CAD build for the part. Positions are in the model's coordinates, mm. Face numbers are marked on the shaded views. A direction names the side the tool comes from. Round coordinates to 2 decimals unless told otherwise and drop trailing zeros. Order: outer loops, then holes, each group sorted by start corner. A loop starts at its lowest first (then second) coordinate and runs counter-clockwise, first axis right, second up. Notation, with made-up numbers: (59, 37.25) -> (105, 37.25) arc R17 ccw to (105, 67.25) -> close; hole circle Ø7 at (71, 10.5). An arc over 180 degrees is marked (long way). Return JSON: item names as keys, results as strings. Group by question number.
Q1. Cut at B-B (x = 18.5). Write the cut outline in (y, z).
Q2. Flat gauge pins, fed straight in: pin 1 (4 mm diameter, centred on y = 13, z = 17.5, fed in from -X); pin 2 (6.5 mm diameter, centred on x = -7, z = 25.5, fed in from -Y); pin 3 (4 mm diameter, centred on x = 28.5, z = 26.5, fed in from -Y). Where does each tip first touch, or does it go through?
Q3. Which spindle directions (+Z, -Z, +X, -X, +Y, -Y) get a long thin tool onto all of the face, cutting with end or side? Do the marked faces 4, 5 and 6. Say none if no direction does.
Q4. Mould opens along Y. For the marked faces 1, 2 and 3 say: +Y half, -Y half, draft (parallel to the pull), parting line (faces both ways), or undercut.
Q5. Cut at A-A (y = 0). Write the cut outline in (x, z), then the cut area to 3 significant figures.
Q6. Cut at D-D (x = -4). Count the separate pieces of the cut face and the enclosed holes in it, then the cut area to 3 significant figures.
Q7. Probe line 1 along Y through (x, z) = (0, 29); line 2 along Y through (x, z) = (0, 54); line 3 along Z through (x, y) = (4.5, -5). List the from-to ranges inside material, lowest first.
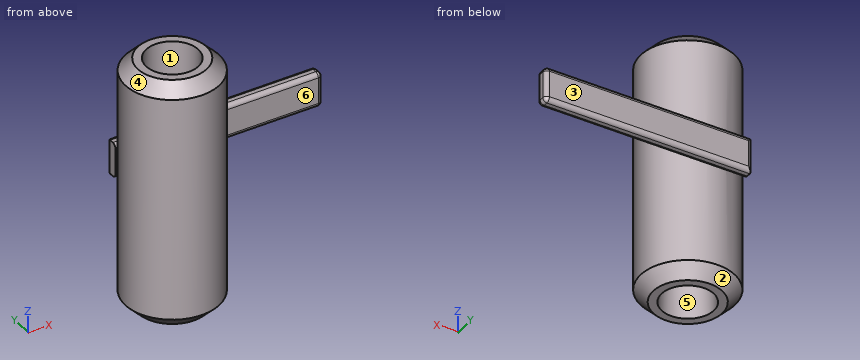
from build123d import *

# Parameters (mm, degrees)
F0_R          = 7.9375
F0_R_2        = 6.35
F2_DEPTH      = 50.8
F3_R          = 14.2875
F3_R_2        = 7.9375
F4_DEPTH      = 63.5
F4_DEPTH_BACK = 12.7
F5_SIZE       = 3.81
F7_START      = -13.97
F6_W          = 64.1522035003
F6_H          = 10.4847997427
F7_DEPTH      = 3.81
F8_T1_DEPTH   = 66.0572035003
F8_T3_DEPTH   = 16.8347997427
F8_T5_DEPTH   = 7.9447997427
F8_T7_DEPTH   = 1.27
F8_S11_W      = 1.27
F8_S11_H      = 1.27
F8_T12_DEPTH  = 1.27
F8_S17_W      = 1.27
F8_S17_H      = 1.27
F8_T18_DEPTH  = 1.27
F8_S23_W      = 1.27
F8_S23_H      = 1.27
F8_T24_DEPTH  = 1.27
F8_S29_W      = 1.27
F8_S29_H      = 1.27
F8_T30_DEPTH  = 1.27
F8_T36_DEPTH  = 54.3607688419
F8_S37_R      = 14.2875
F8_T38_DEPTH  = 29
F8_T42_DEPTH  = 54.3607688419
F8_S43_R      = 14.2875
F8_T44_DEPTH  = 29
F8_T48_DEPTH  = 12.0558566395
F8_S49_R      = 14.2875
F8_T50_DEPTH  = 8
F8_T54_DEPTH  = 12.0558566395
F8_S55_R      = 14.2875
F8_T56_DEPTH  = 8


# Not quite as in the source:
# - a fillet or chamfer that OpenCascade refuses, or shapes differently, is made with other operations: its cross-section is extruded or revolved along the edge and cut away or added
# - a feature names something its author has since deleted; it is built from what else it names


with BuildPart() as f2:
    # F0 (on Top) → F2 (new body)
    with BuildSketch(Plane.XY):
        Circle(F0_R)
        Circle(F0_R_2, mode=Mode.SUBTRACT)
    extrude(amount=F2_DEPTH)

    # F3 (on face) → F4 (join, two sides)
    with BuildSketch(Plane.XY) as f4_sk:
        Circle(F3_R)
        Circle(F3_R_2, mode=Mode.SUBTRACT)
    extrude(amount=F4_DEPTH)
    extrude(f4_sk.sketch, amount=-F4_DEPTH_BACK)

    # F5
    f5_edges = [f2.edges().sort_by_distance(p)[0] for p in [
        (-14.2875, 0, 63.5),
        (-14.2875, 0, -12.7),
    ]]
    chamfer(f5_edges, length=F5_SIZE)

    # F6 (on Front) → F7 (join)
    with BuildSketch(Plane.XZ.offset(F7_START)):
        with Locations((23.3749561012, 26.5372619033)):
            Rectangle(F6_W, F6_H)
    extrude(amount=-F7_DEPTH)

    # F8: fillet of radius 1.27 on 11 edges, made by hand

    # F8_s2 → F8_t1 (cut)
    with BuildSketch(Plane.YZ.offset(-11.876145649)):
        with BuildLine():
            ThreePointArc((16.51, 31.7796617746), (17.4080256121, 31.4076873867), (17.78, 30.5096617746))
            Line((17.78, 30.5096617746), (17.78, 31.7796617746))
            Line((17.78, 31.7796617746), (16.51, 31.7796617746))
        make_face()
        with BuildLine():
            ThreePointArc((16.51, 21.2948620319), (17.4080256121, 21.6668364198), (17.78, 22.5648620319))
            Line((17.78, 22.5648620319), (17.78, 21.2948620319))
            Line((17.78, 21.2948620319), (16.51, 21.2948620319))
        make_face()
    extrude(amount=F8_T1_DEPTH, mode=Mode.SUBTRACT)

    # F8_s4 → F8_t3 (cut)
    with BuildSketch(Plane.XY.offset(18.1198620319)):
        with BuildLine():
            ThreePointArc((-7.431145649, 17.78), (-8.3291712611, 17.4080256121), (-8.701145649, 16.51))
            Line((-8.701145649, 16.51), (-8.701145649, 17.78))
            Line((-8.701145649, 17.78), (-7.431145649, 17.78))
        make_face()
    extrude(amount=F8_T3_DEPTH, mode=Mode.SUBTRACT)

    # F8_s6 → F8_t5 (cut)
    with BuildSketch(Plane.XY.offset(22.5648620319)):
        with BuildLine():
            ThreePointArc((54.1810578513, 13.97), (55.0790834634, 14.3419743879), (55.4510578513, 15.24))
            Line((55.4510578513, 15.24), (55.4510578513, 13.97))
            Line((55.4510578513, 13.97), (54.1810578513, 13.97))
        make_face()
        with BuildLine():
            ThreePointArc((55.4510578513, 16.51), (55.0790834634, 17.4080256121), (54.1810578513, 17.78))
            Line((54.1810578513, 17.78), (55.4510578513, 17.78))
            Line((55.4510578513, 17.78), (55.4510578513, 16.51))
        make_face()
    extrude(amount=F8_T5_DEPTH, mode=Mode.SUBTRACT)

    # F8_s8 → F8_t7 (cut)
    with BuildSketch(Plane.XZ.offset(-16.51)):
        with BuildLine():
            ThreePointArc((54.1810578513, 31.7796617746), (55.0790834634, 31.4076873867), (55.4510578513, 30.5096617746))
            Line((55.4510578513, 30.5096617746), (55.4510578513, 31.7796617746))
            Line((55.4510578513, 31.7796617746), (54.1810578513, 31.7796617746))
        make_face()
        with BuildLine():
            ThreePointArc((54.1810578513, 21.2948620319), (55.0790834634, 21.6668364198), (55.4510578513, 22.5648620319))
            Line((55.4510578513, 22.5648620319), (55.4510578513, 21.2948620319))
            Line((55.4510578513, 21.2948620319), (54.1810578513, 21.2948620319))
        make_face()
    extrude(amount=F8_T7_DEPTH, mode=Mode.SUBTRACT)


with BuildPart() as f8_tool10:
    # F8_s11 → F8_t12 (new body)
    with BuildSketch(Plane.XY.offset(30.5096617746)):
        with Locations((54.8160578513, 17.145)):
            Rectangle(F8_S11_W, F8_S11_H)
    extrude(amount=F8_T12_DEPTH)

    # F8_s13 → F8_t14 (revolve, cut)
    with BuildSketch(Plane(origin=(54.1810578513, 16.51, 30.5096617746), x_dir=(-0.7071067812, -0.7071067812, 0), z_dir=(-0.7071067812, 0.7071067812, 0))):
        with BuildLine():
            ThreePointArc((0, -1.27), (1.27, 0), (0, 1.27))
            Line((0, 1.27), (0, -1.27))
        make_face()
    revolve(axis=Axis((54.1810578513, 16.51, 30.5096617746), (0, 0, 1)), mode=Mode.SUBTRACT)


with BuildPart() as f2_1:
    add(f2.part)

    # F8_t9: cut F8_tool10
    add(f8_tool10.part, mode=Mode.SUBTRACT)


with BuildPart() as f8_tool16:
    # F8_s17 → F8_t18 (new body)
    with BuildSketch(Plane.YZ.offset(54.1810578513)):
        with Locations((17.145, 21.9298620319)):
            Rectangle(F8_S17_W, F8_S17_H)
    extrude(amount=F8_T18_DEPTH)

    # F8_s19 → F8_t20 (revolve, cut)
    with BuildSketch(Plane(origin=(54.1810578513, 16.51, 22.5648620319), x_dir=(0, -0.7071067812, 0.7071067812), z_dir=(0, 0.7071067812, 0.7071067812))):
        with BuildLine():
            ThreePointArc((0, -1.27), (1.27, 0), (0, 1.27))
            Line((0, 1.27), (0, -1.27))
        make_face()
    revolve(axis=Axis((54.1810578513, 16.51, 22.5648620319), (1, 0, 0)), mode=Mode.SUBTRACT)


with BuildPart() as f2_2:
    add(f2_1.part)

    # F8_t15: cut F8_tool16
    add(f8_tool16.part, mode=Mode.SUBTRACT)


with BuildPart() as f8_tool22:
    # F8_s23 → F8_t24 (new body)
    with BuildSketch(Plane.YZ.offset(54.1810578513)):
        with Locations((14.605, 21.9298620319)):
            Rectangle(F8_S23_W, F8_S23_H)
    extrude(amount=F8_T24_DEPTH)

    # F8_s25 → F8_t26 (revolve, cut)
    with BuildSketch(Plane(origin=(54.1810578513, 15.24, 22.5648620319), x_dir=(0, 0.7071067812, 0.7071067812), z_dir=(0, 0.7071067812, -0.7071067812))):
        with BuildLine():
            ThreePointArc((0, -1.27), (1.27, 0), (0, 1.27))
            Line((0, 1.27), (0, -1.27))
        make_face()
    revolve(axis=Axis((54.1810578513, 15.24, 22.5648620319), (1, 0, 0)), mode=Mode.SUBTRACT)


with BuildPart() as f2_3:
    add(f2_2.part)

    # F8_t21: cut F8_tool22
    add(f8_tool22.part, mode=Mode.SUBTRACT)


with BuildPart() as f8_tool28:
    # F8_s29 → F8_t30 (new body)
    with BuildSketch(Plane.XY.offset(30.5096617746)):
        with Locations((54.8160578513, 14.605)):
            Rectangle(F8_S29_W, F8_S29_H)
    extrude(amount=F8_T30_DEPTH)

    # F8_s31 → F8_t32 (revolve, cut)
    with BuildSketch(Plane(origin=(54.1810578513, 15.24, 30.5096617746), x_dir=(-0.7071067812, 0.7071067812, 0), z_dir=(0.7071067812, 0.7071067812, 0))):
        with BuildLine():
            ThreePointArc((0, -1.27), (1.27, 0), (0, 1.27))
            Line((0, 1.27), (0, -1.27))
        make_face()
    revolve(axis=Axis((54.1810578513, 15.24, 30.5096617746), (0, 0, 1)), mode=Mode.SUBTRACT)


with BuildPart() as f2_4:
    add(f2_3.part)

    # F8_t27: cut F8_tool28
    add(f8_tool28.part, mode=Mode.SUBTRACT)


with BuildPart() as f8_tool34:
    # F8_s35 → F8_t36 (new body)
    with BuildSketch(Plane.YZ.offset(-0.1797109906)):
        with BuildLine():
            ThreePointArc((13.97, 22.5648620319), (14.3419743879, 21.6668364198), (15.24, 21.2948620319))
            Line((15.24, 21.2948620319), (13.97, 21.2948620319))
            Line((13.97, 21.2948620319), (13.97, 22.5648620319))
        make_face()
    extrude(amount=F8_T36_DEPTH)

    # F8_s37 → F8_t38 (cut, symmetric)
    with BuildSketch(Plane.XY.offset(21.9)):
        Circle(F8_S37_R)
    extrude(amount=F8_T38_DEPTH, both=True, mode=Mode.SUBTRACT)


with BuildPart() as f2_5:
    add(f2_4.part)

    # F8_t33: cut F8_tool34
    add(f8_tool34.part, mode=Mode.SUBTRACT)


with BuildPart() as f8_tool40:
    # F8_s41 → F8_t42 (new body)
    with BuildSketch(Plane.YZ.offset(54.1810578513)):
        with BuildLine():
            ThreePointArc((13.97, 30.5096617746), (14.3419743879, 31.4076873867), (15.24, 31.7796617746))
            Line((15.24, 31.7796617746), (13.97, 31.7796617746))
            Line((13.97, 31.7796617746), (13.97, 30.5096617746))
        make_face()
    extrude(amount=-F8_T42_DEPTH)

    # F8_s43 → F8_t44 (cut, symmetric)
    with BuildSketch(Plane.XY.offset(31.1)):
        Circle(F8_S43_R)
    extrude(amount=F8_T44_DEPTH, both=True, mode=Mode.SUBTRACT)


with BuildPart() as f2_6:
    add(f2_5.part)

    # F8_t39: cut F8_tool40
    add(f8_tool40.part, mode=Mode.SUBTRACT)


with BuildPart() as f8_tool46:
    # F8_s47 → F8_t48 (new body)
    with BuildSketch(Plane.YZ.offset(-11.876145649)):
        with BuildLine():
            ThreePointArc((15.24, 21.2948620319), (14.3419743879, 21.6668364198), (13.97, 22.5648620319))
            Line((13.97, 22.5648620319), (13.97, 21.2948620319))
            Line((13.97, 21.2948620319), (15.24, 21.2948620319))
        make_face()
    extrude(amount=F8_T48_DEPTH)

    # F8_s49 → F8_t50 (cut, symmetric)
    with BuildSketch(Plane.XY.offset(21.9)):
        Circle(F8_S49_R)
    extrude(amount=F8_T50_DEPTH, both=True, mode=Mode.SUBTRACT)


with BuildPart() as f2_7:
    add(f2_6.part)

    # F8_t45: cut F8_tool46
    add(f8_tool46.part, mode=Mode.SUBTRACT)


with BuildPart() as f8_tool52:
    # F8_s53 → F8_t54 (new body)
    with BuildSketch(Plane.YZ.offset(0.1797109906)):
        with BuildLine():
            ThreePointArc((13.97, 30.5096617746), (14.3419743879, 31.4076873867), (15.24, 31.7796617746))
            Line((15.24, 31.7796617746), (13.97, 31.7796617746))
            Line((13.97, 31.7796617746), (13.97, 30.5096617746))
        make_face()
    extrude(amount=-F8_T54_DEPTH)

    # F8_s55 → F8_t56 (cut, symmetric)
    with BuildSketch(Plane.XY.offset(31.1)):
        Circle(F8_S55_R)
    extrude(amount=F8_T56_DEPTH, both=True, mode=Mode.SUBTRACT)


with BuildPart() as f2_8:
    add(f2_7.part)

    # F8_t51: cut F8_tool52
    add(f8_tool52.part, mode=Mode.SUBTRACT)


solid = f2_8.part
Solution:
{
 "1": {"outline": "(13.97, 22.56) arc R1.27 ccw to (15.24, 21.29) -> (16.51, 21.29) arc R1.27 ccw to (17.78, 22.56) -> (17.78, 30.51) arc R1.27 ccw to (16.51, 31.78) -> (15.24, 31.78) arc R1.27 ccw to (13.97, 30.51) -> close"},
 "2": {"pin 1": "stops at x = -9.12", "pin 2": "stops at y = -13.79", "pin 3": "stops at y = 13.97"},
 "3": {"face 4": "+Z", "face 5": "-Z", "face 6": "+Z, -Z, +X"},
 "4": {"face 1": "undercut", "face 2": "parting line", "face 3": "+Y half"},
 "5": {"outline": "(-14.29, -8.89) -> (-10.48, -12.7) -> (-7.94, -12.7) -> (-7.94, 0) -> (-6.35, 0) -> (-6.35, 50.8) -> (-7.94, 50.8) -> (-7.94, 63.5) -> (-10.48, 63.5) -> (-14.29, 59.69) -> close; (6.35, 0) -> (7.94, 0) -> (7.94, -12.7) -> (10.48, -12.7) -> (14.29, -8.89) -> (14.29, 59.69) -> (10.48, 63.5) -> (7.94, 63.5) -> (7.94, 50.8) -> (6.35, 50.8) -> close", "area": "1,100 mm²"},
 "6": {"separate pieces": "3", "enclosed holes": "0", "area": "1,250 mm²"},
 "7": {"line 1": "y = -14.29 to -6.35, 6.35 to 17.78", "line 2": "y = -14.29 to -7.94, 7.94 to 14.29", "line 3": "z = 0 to 50.8"}
}
